Geometry: final body of the model. Coordinates: model frame, mm. Face numbers are marked on the shaded views. A direction names the side the tool comes from. Coordinates: 2 decimals unless noted, no trailing zeros. Write each loop counter-clockwise with the first axis right and the second up, starting at its lowest first coordinate (ties: lowest second). Pieces come first, ordered by that corner, then holes.
from build123d import *

# Parameters (mm, degrees)
SKETCH1_R           = 1.1
BOSS_EXTRUDE1_DEPTH = 6
SKETCH2_W           = 2
SKETCH2_H           = 2
BOSS_EXTRUDE2_DEPTH = 16
SKETCH4_W           = 2
SKETCH4_H           = 11.994112908
BOSS_EXTRUDE4_DEPTH = 19
SKETCH5_W           = 1
SKETCH5_H           = 1
BOSS_EXTRUDE5_DEPTH = 2.5
SKETCH6_W           = 1
SKETCH6_H           = 1.25
BOSS_EXTRUDE6_DEPTH = 6
SKETCH7_W           = 3.009444154
SKETCH7_H           = 11.994112908
BOSS_EXTRUDE7_DEPTH = 7
SKETCH8_R           = 1.1
BOSS_EXTRUDE8_DEPTH = 1
SKETCH9_R           = 1.1
CUT_EXTRUDE1_DEPTH  = 10
SKETCH10_W          = 19
SKETCH10_H          = 9.734535385
CUT_EXTRUDE2_DEPTH  = 10


with BuildPart() as part:
    # Sketch1 → Boss-Extrude1 (new body)
    with BuildSketch(Plane.XY):
        with BuildLine():
            Line((0, -24.3), (0, -30.3))
            Line((0, -30.3), (6, -30.3))
            Line((6, -30.3), (6, -23.547611344))
            ThreePointArc((6, -23.547611344), (3.023495026, -24.111169151), (0, -24.3))
        make_face()
        with Locations((3, -27.152103588)):
            Circle(SKETCH1_R, mode=Mode.SUBTRACT)
    extrude(amount=BOSS_EXTRUDE1_DEPTH)

    # Sketch2 → Boss-Extrude2 (add)
    with BuildSketch(Plane.XZ.offset(30.3)):
        with Locations((2.994992787, 3)):
            Rectangle(SKETCH2_W, SKETCH2_H)
    extrude(amount=BOSS_EXTRUDE2_DEPTH)

    # Sketch4 → Boss-Extrude4 (add)
    with BuildSketch(Plane(origin=(0, 0, 2), x_dir=(-1, 0, 0), z_dir=(0, 0, -1))):
        with Locations((-2.994992787, -40.302943546)):
            Rectangle(SKETCH4_W, SKETCH4_H)
    extrude(amount=BOSS_EXTRUDE4_DEPTH)

    # Sketch5 → Boss-Extrude5 (add)
    with BuildSketch(Plane.XZ.offset(30.3)):
        with Locations((3.093546014, 5.062561083)):
            Rectangle(SKETCH5_W, SKETCH5_H)
    extrude(amount=BOSS_EXTRUDE5_DEPTH)

    # Sketch6 → Boss-Extrude6 (add)
    with BuildSketch(Plane.XY.offset(5.562561083)):
        with Locations((3.093546014, -32.175)):
            Rectangle(SKETCH6_W, SKETCH6_H)
    extrude(amount=BOSS_EXTRUDE6_DEPTH)

    # Sketch7 → Boss-Extrude7 (add)
    with BuildSketch(Plane.ZY.offset(-1.994992787)):
        with Locations((-15.495277923, -40.302943546)):
            Rectangle(SKETCH7_W, SKETCH7_H)
    extrude(amount=BOSS_EXTRUDE7_DEPTH)

    # Sketch8 → Boss-Extrude8 (add)
    with BuildSketch(Plane(origin=(0, 0, 0), x_dir=(-1, 0, 0), z_dir=(0, 0, -1))):
        with Locations((-3, -27.152103588)):
            Circle(SKETCH8_R)
    extrude(amount=-BOSS_EXTRUDE8_DEPTH)

    # Sketch9 → Cut-Extrude1 (cut)
    with BuildSketch(Plane.XY.offset(6)):
        with Locations((3, -27.152103588)):
            Circle(SKETCH9_R)
    extrude(amount=-CUT_EXTRUDE1_DEPTH, mode=Mode.SUBTRACT)

    # Sketch10 → Cut-Extrude2 (cut)
    with BuildSketch(Plane.ZY.offset(5.005007213)):
        with Locations((-7.5, -39.173154784)):
            Rectangle(SKETCH10_W, SKETCH10_H)
    extrude(amount=-CUT_EXTRUDE2_DEPTH, mode=Mode.SUBTRACT)


solid = part.part
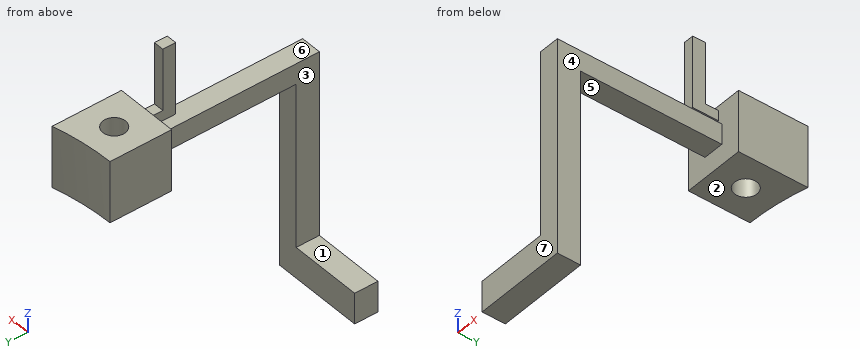
Item 1: Section D-D, the plane y = -26.5. Output: boundary loops of the cut face in (x, z), plus the area to 3 significant figures.
Derived:
outline: (0, 0) - (2.11, 0) - (2.11, 6) - (0, 6) - close; (3.89, 0) - (6, 0) - (6, 6) - (3.89, 6) - close
area: 25.4 mm2
Item 2: Material intervals for probe 1 along Z at (x, y) = (3.5, -31.25); probe 2 along Y at (x, z) = (3, 1.9); probe 3 along Z at (x, y) = (1.25, -29.75), sorted ascending.
Derived:
probe 1: z = 2 to 4, 4.56 to 5.56
probe 2: y = -46.3 to -44.04, -30.3 to -28.25, -26.05 to -24.11
probe 3: z = 0 to 6
Item 3: Section B-B, the plane y = -32. Output: boundary loops of the cut face in (x, z) (3 decimals), plus the area to 3 significant figures.
Derived:
outline: (1.995, 2) - (3.995, 2) - (3.995, 4) - (1.995, 4) - close; (2.594, 4.563) - (3.594, 4.563) - (3.594, 11.563) - (2.594, 11.563) - close
area: 11.0 mm2
Item 4: Section C-C, the plane z = -15. Output: boundary loops of the cut face in (x, y) (3 decimals), plus the area to 3 significant figures.
Derived:
outline: (-5.005, -46.3) - (3.995, -46.3) - (3.995, -44.04) - (-5.005, -44.04) - close
area: 20.3 mm2
Item 5: Set-up query: the marked faces 1, 2, 3 and 4. Return all of +Z, -Z, +X, -X, +Y, -Y with unobstructed straight access to the full face (end or side cutting, diameter ignored); none if empty.
Derived:
face 1: +Z, -X, +Y, -Y
face 2: -Z, +X, -X, +Y
face 3: +Z, -X, -Y
face 4: +Z, -Z, +X, -Y
Item 6: Pull-direction query (Y, two-part tool) for the marked faces 5, 6 and 7; classes: released by +Y, released by -Y, zero draft, split by the parting line, or undercut.
Derived:
face 5: undercut
face 6: zero draft
face 7: released by -Y
Item 7: Pin query (flat end, axial travel): pin 1 (13 mm diameter, centred on y = -40.5, z = -4.5, fed in from +X) (3 decimals); pin 2 (0.5 mm diameter, centred on x = 3, y = -31, fed in from +Z); pin 3 (1.8 mm diameter, centred on x = 3.5, y = -27, fed in from -Z). Return the tip coordinate at first contact, or that it passes through.
Derived:
pin 1: stops at x = 3.995
pin 2: stops at z = 5.56
pin 3: stops at z = 0
Item 8: Section A-A, the plane x = 3. Output: boundary loops of the cut face in (y, z).
Derived:
outline: (-46.3, -17) - (-44.04, -17) - (-44.04, 2) - (-30.3, 2) - (-30.3, 0) - (-28.25, 0) - (-28.25, 6) - (-30.3, 6) - (-30.3, 5.56) - (-31.55, 5.56) - (-31.55, 11.56) - (-32.8, 11.56) - (-32.8, 4.56) - (-30.3, 4.56) - (-30.3, 4) - (-46.3, 4) - close; (-26.05, 0) - (-24.11, 0) - (-24.11, 6) - (-26.05, 6) - close
